Study the drawing (mm; zero at the part's minimum x, y, z) and answer. Round coordinates to 2 decimals unless told otherwise and drop trailing zeros. Write each loop counter-clockwise with the first axis right and the second up, starting at its lowest first coordinate (ties: lowest second). Pieces come first, ordered by that corner, then holes. Notation, with made-up numbers: (2.25, 89) -> (12.25, 89) arc R22 cw to (12.25, 112) -> close; hole circle Ø6 at (62.25, 11). An arc over 180 degrees is marked (long way). Return JSON: item names as keys, results as strings.
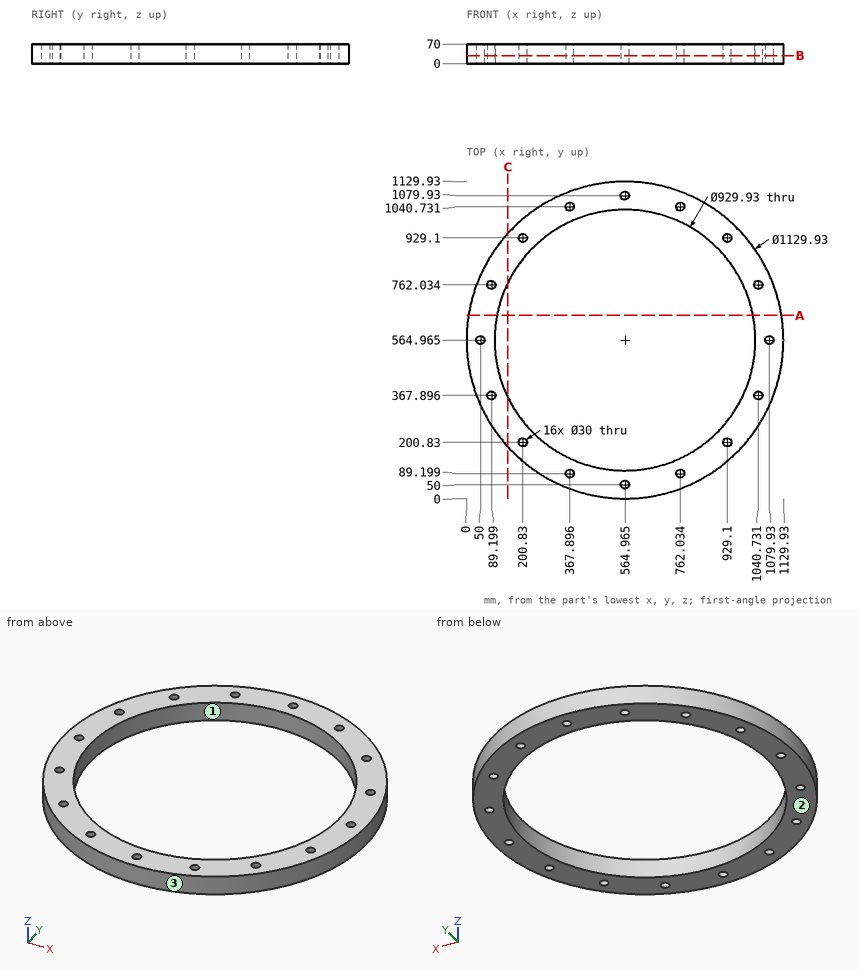
Item 1: Section B-B (z = 29) is taken. State how many separate pieces and enclosed holes the cut face has, then the cut area to 3 significant figures.
Worked answers:
{"separate pieces": "1", "enclosed holes": "17", "area": "312,000 mm2"}
Item 2: Section C-C (x = 147.5) is taken. Give the vertices of the cut face in (y, z), then the cut area to 3 significant figures.
Worked answers:
{"outline": "(184.3, 0) -> (360.23, 0) -> (360.23, 70) -> (184.3, 70) -> close; (769.7, 0) -> (945.63, 0) -> (945.63, 70) -> (769.7, 70) -> close", "area": "24,600 mm2"}
Item 3: For a pull along X with two mould halves and no side action, classify the marked faces 1, 2 and 3 as released by +X, released by -X, zero draft, split by the parting line, or undercut.
Worked answers:
{"face 1": "undercut", "face 2": "zero draft", "face 3": "split by the parting line"}
Item 4: Straight lines are drawn through the part: L1, parallel to Y at x = 568, z = 26; L2, parallel to X at y = 380, z = 66 (1 decimal); L3, parallel to Y at x = 932, z = 22 (1 decimal). For each, find the intervals that lie inside material, in ascending order. Write a range as [from, to].
Worked answers:
{"L1": "y = [0.01, 35.31], [64.69, 100.01], [1029.92, 1065.24], [1094.62, 1129.92]", "L2": "x = [31.1, 80.3], [98.1, 138.4], [991.6, 1031.9], [1049.6, 1098.8]", "L3": "y = [135.5, 186.1], [215.5, 279.5], [850.4, 914.4], [943.8, 994.5]"}
Item 5: Section A-A (y = 653.5) is taken. Give the vertices of the cut face in (x, z).
Worked answers:
{"outline": "(6.98, 0) -> (108.51, 0) -> (108.51, 70) -> (6.98, 70) -> close; (1021.42, 0) -> (1122.95, 0) -> (1122.95, 70) -> (1021.42, 70) -> close"}
Item 6: Flat-ended cylindrical pins translate along their axes: pin 1 (18 mm diameter, centred on x = 1040.73, y = 367.9, fed in from +Z); pin 2 (6 mm diameter, centred on y = 985, z = 20, fed in from -X) (1 decimal); pin 3 (3 mm diameter, centred on y = 322.5, z = 21.5, fed in from -X) (1 decimal); pin 4 (1 mm diameter, centred on y = 672, z = 16.5, fed in from +X) (1 decimal). Find the tip coordinate at first contact, or state that the pin passes through.
Worked answers:
{"pin 1": "passes through", "pin 2": "stops at x = 183.8", "pin 3": "stops at x = 54", "pin 4": "stops at x = 1119.8"}
